CAD build for the part. Positions are in the model's coordinates, mm. Face numbers are marked on the shaded views. Coordinates: 2 decimals unless noted, no trailing zeros. Order: outer loops, then holes, each group sorted by start corner. A loop starts at its lowest first (then second) coordinate and runs counter-clockwise, first axis right, second up. Notation, with made-up numbers: (86.25, -5) - (113.25, -5) arc R30 ccw to (113.25, 25) - close; hole circle Ø1 at (77.25, 66.5). An arc over 180 degrees is marked (long way). Return JSON: item names as keys, results as strings.
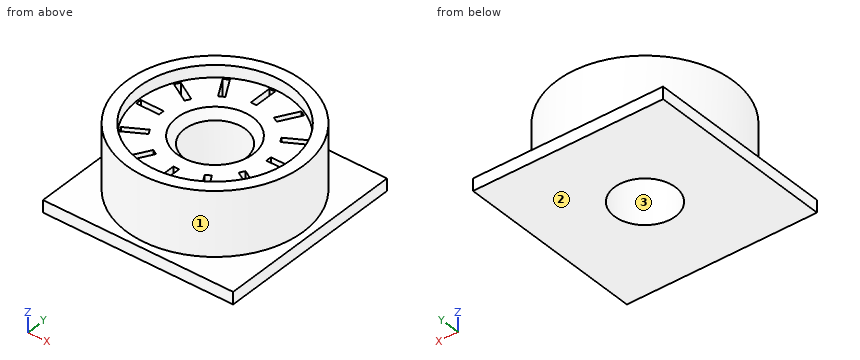
Autodesk Fusion 360 part; units mm, degrees
sketch "Sketch1" plane through (0, 0, 0) normal (0, 1, 0) x (1, 0, 0)
  line L0 (0, 0) -> (11.6, 0)
  line L1 (11.6, 0) -> (11.6, -10)
  line L2 (11.6, -10) -> (0, -10)
  line L3 (0, -10) -> (0, 0)
  line L4 (10, -10) -> (0, -10)
  line L5 (0, -10) -> (0, -8.4)
  line L6 (0, -8.4) -> (10, -8.4)
  line L7 (10, -8.4) -> (10, -10)
  line L8 (4, -8.4) -> (0, -8.4)
  line L9 (0, -8.4) -> (0, 0)
  line L10 (0, 0) -> (4, 0)
  line L11 (4, 0) -> (4, -8.4)
  line L12 (4, -7.4) -> (5, -8.4)
  dimension "d1" = 1.6
  dimension "d2" = 1.6
  dimension "d3" = 10
  dimension "d5" = 8.4
  dimension "d6" = 4
  dimension "d8" = 1
  dimension "d9" = 45
revolve "Revolve1" add sketch "Sketch1" angle 360 about axis through (0, 0, 10) along (0, 0, -1) contours L0 L1 L2 L6 L7 L11 L12
sketch "Sketch2" plane through (0, 0, 0) normal (0, 0, -1) x (1, 0, 0)
  circle A0 centre (0, 0) radius 4
  circle A1 centre (0, 0) radius 11.6
  line L0 (-12.5, 12.5) -> (12.5, 12.5)
  line L1 (12.5, 12.5) -> (12.5, -12.5)
  line L2 (12.5, -12.5) -> (-12.5, -12.5)
  line L3 (-12.5, -12.5) -> (-12.5, 12.5)
  line L4 (-12.5, 12.5) -> (12.5, -12.5) construction
  line L5 (12.5, 12.5) -> (-12.5, -12.5) construction
  dimension "d10" = 25
extrude "Extrude1" add sketch "Sketch2" against normal blind 1.6 contours L0 L1 L2 L3
sketch "Sketch3" plane through (0, 0, 8.4) normal (0, 0, 1) x (-1, 0, 0)
  circle A0 centre (0, 0) radius 10
  circle A1 centre (0, 0) radius 5
  line L0 (9.75, 0) -> (6.75, 0)
  line L1 (6.75, 0) -> (6.75, 0.75)
  line L2 (6.75, 0.75) -> (9.75, 0.75)
  line L3 (9.75, 0.75) -> (9.75, 0)
  dimension "d13" = 3
  dimension "d14" = 6.75
  dimension "d15" = 0.75
extrude "Extrude2" cut sketch "Sketch3" against normal blind 4.4 contours L0 L1 L2 L3
pattern_circular "C-Pattern1" count 12 over 360 about axis through (0, 0, 0) along (0, 0, 1) of "Extrude2"
Item 1: Wall check: L1, parallel to Y at x = 0, z = 2.75; L2, parallel to Y at x = 0, z = 9.45. Give the ranges that are in metal, low to high. Write a range as [from, to].
Findings below:
{"L1": "y = [-11.6, -4], [4, 11.6]", "L2": "y = [-11.6, -10], [10, 11.6]"}
Item 2: Band-saw the part on B-B, the plane z = 3. List the corners of the cut face in (x, y), then the cut area to 3 significant figures.
Findings below:
{"outline": "circle Ø23.2 at (0, 0); hole circle Ø8 at (0, 0)", "area": "372 mm²"}
Item 3: Mould opens along X. For the marked faces 1, 2 and 3 say: released by +X, released by -X, zero draft, split by the parting line, or undercut.
Findings below:
{"face 1": "split by the parting line", "face 2": "zero draft", "face 3": "undercut"}
Item 4: Band-saw the part on A-A, the plane x = 7.75. List the corners of the cut face in (y, z), then the cut area to 3 significant figures.
Findings below:
{"outline": "(-12.5, 0) - (12.5, 0) - (12.5, 1.6) - (8.63, 1.6) - (8.63, 10) - (6.32, 10) - (6.32, 8.4) - (5.34, 8.4) - (5.34, 4) - (4.47, 4) - (4.47, 8.4) - (0.75, 8.4) - (0.75, 4) - (0, 4) - (0, 8.4) - (-3.61, 8.4) - (-3.61, 4) - (-4.47, 4) - (-4.47, 8.4) - (-6.32, 8.4) - (-6.32, 10) - (-8.63, 10) - (-8.63, 1.6) - (-12.5, 1.6) - close", "area": "154 mm²"}
Item 5: Drop flat-ended pins along their axis: P1, Ø0.8, axis at y = -0.5, z = 6.5, coming from the +X side; P2, Ø0.8, axis at x = -0.5, z = 6.5, coming from the +Y side; P3, Ø1.1, axis at x = -4.5, y = 7, coming from the +Z side. Give the stop position or say it passes through.
Findings below:
{"P1": "stops at x = 11.6", "P2": "stops at y = 11.6", "P3": "stops at z = 8.4"}
